Autodesk Inventor part; units mm, degrees
ref_plane "YZ Plane" through (0, 0, 0) normal (1, 0, 0) x (0, 1, 0)
ref_plane "XZ Plane" through (0, 0, 0) normal (0, 1, 0) x (-1, 0, 0)
ref_plane "XY Plane" through (0, 0, 0) normal (0, 0, 1) x (1, 0, 0)
sketch "Sketch1" plane through (0, 0, 0) normal (0, 1, 0) x (-1, 0, 0)
  line L0 (0, 0) -> (0, 27) construction
  line L1 (0, 0) -> (0, 1.2679)
  line L2 (0, 4.7321) -> (0, 22.2679)
  line L3 (0, 27) -> (0, 25.7321)
  line L4 (-1, 30.1625) -> (-1, -2.7373)
  line L5 (0, 27) -> (-1, 27)
  line L6 (0, 0) -> (-1, 0)
  line L7 (0, 26) -> (0, 22) construction
  line L8 (0, 24) -> (-1, 24) construction
  circle A0 centre (-1, 24) radius 2
  line L9 (0, 5) -> (0, 1) construction
  line L10 (0, 3) -> (-1, 3) construction
  circle A1 centre (-1, 3) radius 2
  dimension "d0" = 27
  dimension "d8" = 1
  dimension "d9" = 4
  dimension "d10" = 4
revolve "Revolution1" add sketch "Sketch1" angle 360 about axis through (1, 0, 30.1625) along (0, 0, -1) picked at (-0.5539, 3.4954) picked at (-0.772, 24.6265) contours L6 L4 A1 L1 | A1 L4 | A1 L4 A0 L2 | A0 L4 | L4 L5 L3 A0
properties part number "Delts Robot Arm Joint Rod"
Can you work these out from the model? Positions are in its coordinate system, mm. A direction names the side the tool comes from. Round coordinates to 2 decimals unless told otherwise and drop trailing zeros. Loops run counter-clockwise (first coordinate to the right, second up) from the corner with the lowest first, then second, coordinate; pieces in that order, holes last.
Item 1: Please list where these lines run through material, in increasing order: L1, parallel to Y at x = 1.1, z = 5; L2, parallel to Z at x = 2.2, y = -0.9; L3, parallel to Z at x = 0.65, y = -1.3.
Item 2: Suppose I cut it at C-C, the plane x = 0.75. Write out the boundary of the cut face in (y, z).
Item 3: If we mould it in two halves opening along Z, with no side actions, what happens to faces 1 (the flat face through (1, 0, 0)), 2 (the cylindrical face through (1, -1, 26)), 3 (the cylindrical face through (1, 1, 14))? For each: +Z half, -Z half, draft (parallel to the pull), parting line (faces both ways), or undercut.
Item 4: Will these pins go through, and if not, where does the flat tip stop? pin 1 Ø1 at (x, z) = (1.5, 5) entering from +Y; pin 2 Ø2 at (x, z) = (0.5, 8.5) entering from +Y.
Item 5: Suppose I cut it at D-D, the plane y = -1.4. Write out the boundary of the cut face in (x, z).
Item 6: Suppose I cut it at B-B, the plane y = -0.4. Write out the boundary of the cut face in (x, z).
Item 7: Which directions (+Z, -Z, +X, -X, +Y, -Y) give clear straight access to the entire face, cutting with the end or side of a thin tool? Please do faces 4 (the flat face through (1, 0, 27)), 5 (the cylindrical face through (1, 1, 1)).
Item 8: Suppose I cut it at A-A, the plane x = 2.6. Write out the boundary of the cut face in (y, z).
Reported:
1. L1: y = -0.99 to 0.99
1. L2: z = 1.68 to 4.32, 22.68 to 25.32
1. L3: z = 1.52 to 4.48, 22.52 to 25.48
2. outline: (-0.97, 0) - (0.97, 0) - (0.97, 1.27) arc R1.98 ccw to (0.97, 4.73) - (0.97, 22.27) arc R1.98 ccw to (0.97, 25.73) - (0.97, 27) - (-0.97, 27) - (-0.97, 25.73) arc R1.98 ccw to (-0.97, 22.27) - (-0.97, 4.73) arc R1.98 ccw to (-0.97, 1.27) - close
3. face 1: -Z half
3. face 2: draft
3. face 3: undercut
4. pin 1: stops at y = 1.25
4. pin 2: stops at y = 1
5. outline: circle Ø2.86 at (1, 3); circle Ø2.86 at (1, 24)
6. outline: (0.08, 0) - (1.92, 0) - (1.92, 1.27) arc R1.96 ccw to (1.92, 4.73) - (1.92, 22.27) arc R1.96 ccw to (1.92, 25.73) - (1.92, 27) - (0.08, 27) - (0.08, 25.73) arc R1.96 ccw to (0.08, 22.27) - (0.08, 4.73) arc R1.96 ccw to (0.08, 1.27) - close
7. face 4: +Z, +X, -X, +Y, -Y
7. face 5: -Z
8. outline: circle Ø2.4 at (0, 3); circle Ø2.4 at (0, 24)
